```python
from build123d import *

# Parameters (mm, degrees)
ESQUISSE1_R        = 2.1
BOSS_EXTRU_1_DEPTH = 150


with BuildPart() as part:
    # Esquisse1 → Boss.-Extru.1 (new, symmetric)
    with BuildSketch(Plane.XY):
        with BuildLine():
            Line((-38.199999929, 10), (-34.639999675, 10))
            Line((-34.639999675, 10), (-32.839999603, 8.2))
            Line((-32.839999603, 8.2), (-35.499339671, 8.2))
            Line((-35.499339671, 8.2), (-35.499339671, 6.56))
            Line((-35.499339671, 6.56), (-32.839999603, 3.900660038))
            Line((-32.839999603, 3.900660038), (-27.159999603, 3.900660038))
            Line((-27.159999603, 3.900660038), (-24.500659536, 6.56))
            Line((-24.500659536, 6.56), (-24.500659536, 8.2))
            Line((-24.500659536, 8.2), (-27.159999603, 8.2))
            Line((-27.159999603, 8.2), (-25.359999532, 10))
            Line((-25.359999532, 10), (-14.640000468, 10))
            Line((-14.640000468, 10), (-12.840000397, 8.2))
            Line((-12.840000397, 8.2), (-15.499340464, 8.2))
            Line((-15.499340464, 8.2), (-15.499340464, 6.56))
            Line((-15.499340464, 6.56), (-12.840000397, 3.900660038))
            Line((-12.840000397, 3.900660038), (-7.159998809, 3.900660038))
            Line((-7.159998809, 3.900660038), (-4.500658742, 6.56))
            Line((-4.500658742, 6.56), (-4.500658742, 8.2))
            Line((-4.500658742, 8.2), (-7.159998809, 8.2))
            Line((-7.159998809, 8.2), (-5.359998738, 10))
            Line((-5.359998738, 10), (5.359998738, 10))
            Line((5.359998738, 10), (7.159998809, 8.2))
            Line((7.159998809, 8.2), (4.500658742, 8.2))
            Line((4.500658742, 8.2), (4.500658742, 6.56))
            Line((4.500658742, 6.56), (7.159998809, 3.900660038))
            Line((7.159998809, 3.900660038), (12.840000397, 3.900660038))
            Line((12.840000397, 3.900660038), (15.499340464, 6.56))
            Line((15.499340464, 6.56), (15.499340464, 8.2))
            Line((15.499340464, 8.2), (12.840000397, 8.2))
            Line((12.840000397, 8.2), (14.640000468, 10))
            Line((14.640000468, 10), (25.359999532, 10))
            Line((25.359999532, 10), (27.159999603, 8.2))
            Line((27.159999603, 8.2), (24.500659536, 8.2))
            Line((24.500659536, 8.2), (24.500659536, 6.56))
            Line((24.500659536, 6.56), (27.159999603, 3.900660038))
            Line((27.159999603, 3.900660038), (32.839999603, 3.900660038))
            Line((32.839999603, 3.900660038), (35.499339671, 6.56))
            Line((35.499339671, 6.56), (35.499339671, 8.2))
            Line((35.499339671, 8.2), (32.839999603, 8.2))
            Line((32.839999603, 8.2), (34.639999675, 10))
            Line((34.639999675, 10), (38.199999929, 10))
            ThreePointArc((38.199999929, 10), (39.47279216, 9.472792181), (39.999999929, 8.199999929))
            Line((39.999999929, 8.199999929), (39.999999787, 4.639999675))
            Line((39.999999787, 4.639999675), (38.199999716, 2.839999675))
            Line((38.199999716, 2.839999675), (38.199999821, 5.499339742))
            Line((38.199999821, 5.499339742), (36.559999821, 5.499339807))
            Line((36.559999821, 5.499339807), (33.900659754, 2.839999845))
            Line((33.900659754, 2.839999845), (33.900659641, 0))
            Line((33.900659641, 0), (33.900659754, -2.839999845))
            Line((33.900659754, -2.839999845), (36.559999821, -5.499339807))
            Line((36.559999821, -5.499339807), (38.199999821, -5.499339742))
            Line((38.199999821, -5.499339742), (38.199999716, -2.839999675))
            Line((38.199999716, -2.839999675), (39.999999787, -4.639999675))
            Line((39.999999787, -4.639999675), (39.999999929, -8.199999929))
            ThreePointArc((39.999999929, -8.199999929), (39.47279216, -9.472792181), (38.199999929, -10))
            Line((38.199999929, -10), (34.639999675, -10))
            Line((34.639999675, -10), (32.839999603, -8.2))
            Line((32.839999603, -8.2), (35.499339671, -8.2))
            Line((35.499339671, -8.2), (35.499339671, -6.56))
            Line((35.499339671, -6.56), (32.839999603, -3.900660038))
            Line((32.839999603, -3.900660038), (27.159999603, -3.900660038))
            Line((27.159999603, -3.900660038), (24.500659536, -6.56))
            Line((24.500659536, -6.56), (24.500659536, -8.2))
            Line((24.500659536, -8.2), (27.159999603, -8.2))
            Line((27.159999603, -8.2), (25.359999532, -10))
            Line((25.359999532, -10), (14.640000468, -10))
            Line((14.640000468, -10), (12.840000397, -8.2))
            Line((12.840000397, -8.2), (15.499340464, -8.2))
            Line((15.499340464, -8.2), (15.499340464, -6.56))
            Line((15.499340464, -6.56), (12.840000397, -3.900660038))
            Line((12.840000397, -3.900660038), (7.159998809, -3.900660038))
            Line((7.159998809, -3.900660038), (4.500658742, -6.56))
            Line((4.500658742, -6.56), (4.500658742, -8.2))
            Line((4.500658742, -8.2), (7.159998809, -8.2))
            Line((7.159998809, -8.2), (5.359998738, -10))
            Line((5.359998738, -10), (-5.359998738, -10))
            Line((-5.359998738, -10), (-7.159998809, -8.2))
            Line((-7.159998809, -8.2), (-4.500658742, -8.2))
            Line((-4.500658742, -8.2), (-4.500658742, -6.56))
            Line((-4.500658742, -6.56), (-7.159998809, -3.900660038))
            Line((-7.159998809, -3.900660038), (-12.840000397, -3.900660038))
            Line((-12.840000397, -3.900660038), (-15.499340464, -6.56))
            Line((-15.499340464, -6.56), (-15.499340464, -8.2))
            Line((-15.499340464, -8.2), (-12.840000397, -8.2))
            Line((-12.840000397, -8.2), (-14.640000468, -10))
            Line((-14.640000468, -10), (-25.359999532, -10))
            Line((-25.359999532, -10), (-27.159999603, -8.2))
            Line((-27.159999603, -8.2), (-24.500659536, -8.2))
            Line((-24.500659536, -8.2), (-24.500659536, -6.56))
            Line((-24.500659536, -6.56), (-27.159999603, -3.900660038))
            Line((-27.159999603, -3.900660038), (-32.839999603, -3.900660038))
            Line((-32.839999603, -3.900660038), (-35.499339671, -6.56))
            Line((-35.499339671, -6.56), (-35.499339671, -8.2))
            Line((-35.499339671, -8.2), (-32.839999603, -8.2))
            Line((-32.839999603, -8.2), (-34.639999675, -10))
            Line((-34.639999675, -10), (-38.199999929, -10))
            ThreePointArc((-38.199999929, -10), (-39.47279216, -9.472792181), (-39.999999929, -8.199999929))
            Line((-39.999999929, -8.199999929), (-39.999999787, -4.639999675))
            Line((-39.999999787, -4.639999675), (-38.199999716, -2.839999675))
            Line((-38.199999716, -2.839999675), (-38.199999821, -5.499339742))
            Line((-38.199999821, -5.499339742), (-36.559999821, -5.499339807))
            Line((-36.559999821, -5.499339807), (-33.900659754, -2.839999845))
            Line((-33.900659754, -2.839999845), (-33.900659641, 0))
            Line((-33.900659641, 0), (-33.900659754, 2.839999845))
            Line((-33.900659754, 2.839999845), (-36.559999821, 5.499339807))
            Line((-36.559999821, 5.499339807), (-38.199999821, 5.499339742))
            Line((-38.199999821, 5.499339742), (-38.199999716, 2.839999675))
            Line((-38.199999716, 2.839999675), (-39.999999787, 4.639999675))
            Line((-39.999999787, 4.639999675), (-39.999999929, 8.199999929))
            ThreePointArc((-39.999999929, 8.199999929), (-39.47279216, 9.472792181), (-38.199999929, 10))
        make_face()
        with Locations((-29.999999603, 0)):
            Circle(ESQUISSE1_R, mode=Mode.SUBTRACT)
        with Locations((-9.999999603, 0)):
            Circle(ESQUISSE1_R, mode=Mode.SUBTRACT)
        with Locations(Location((29.999999603, 0, 0), (0, 0, 180))):
            Circle(ESQUISSE1_R, mode=Mode.SUBTRACT)
        with Locations(Location((9.999999603, 0, 0), (0, 0, 180))):
            Circle(ESQUISSE1_R, mode=Mode.SUBTRACT)
        Polygon((-38.199999929, 8.2), (-38.199999864, 6.569339742), (-37.629999799, 6.569339742), (-36.569339648, 7.629999935), (-36.569339648, 8.2), align=None, mode=Mode.SUBTRACT)
        Polygon((-17.3, 6.239339079), (-17.3, 8.2), (-22.7, 8.2), (-22.7, 6.239339079), (-26.099339368, 2.839999845), (-26.099339368, -2.839999845), (-22.7, -6.239339079), (-22.7, -8.2), (-17.3, -8.2), (-17.3, -6.239339079), (-13.900660632, -2.839999845), (-13.900660632, 2.839999845), align=None, mode=Mode.SUBTRACT)
        Polygon((-6.099339678, -2.840000949), (-6.099339678, 2.840000949), (-2.700001413, 6.239339079), (-2.700001413, 8.2), (2.700001413, 8.2), (2.700001413, 6.239339079), (6.099339678, 2.840000949), (6.099339678, -2.840000949), (2.700001413, -6.239339079), (2.700001413, -8.2), (-2.700001413, -8.2), (-2.700001413, -6.239339079), align=None, mode=Mode.SUBTRACT)
        Polygon((-36.569339648, -7.629999935), (-36.569339648, -8.2), (-38.199999929, -8.2), (-38.199999864, -6.569339742), (-37.629999799, -6.569339742), align=None, mode=Mode.SUBTRACT)
        Polygon((36.569339648, 8.2), (38.199999929, 8.2), (38.199999864, 6.569339742), (37.629999799, 6.569339742), (36.569339648, 7.629999935), align=None, mode=Mode.SUBTRACT)
        Polygon((36.569339648, -8.2), (38.199999929, -8.2), (38.199999864, -6.569339742), (37.629999799, -6.569339742), (36.569339648, -7.629999935), align=None, mode=Mode.SUBTRACT)
        Polygon((13.900660632, -2.839999845), (17.3, -6.239339079), (17.3, -8.2), (22.7, -8.2), (22.7, -6.239339079), (26.099339368, -2.839999845), (26.099339368, 2.839999845), (22.7, 6.239339079), (22.7, 8.2), (17.3, 8.2), (17.3, 6.239339079), (13.900660632, 2.839999845), align=None, mode=Mode.SUBTRACT)
    extrude(amount=BOSS_EXTRU_1_DEPTH, both=True)


solid = part.part
```
Part model, mm, in its own coordinate system. A direction names the side the tool comes from. Round coordinates to 2 decimals unless told otherwise and drop trailing zeros. Write each loop counter-clockwise with the first axis right and the second up, starting at its lowest first coordinate (ties: lowest second). Pieces come first, ordered by that corner, then holes. Notation, with made-up numbers: M 72,42 L 81,42 A27 cw 81,74 Z; hole C -14,30.5 d11. An arc over 180 degrees is marked long. One line per question, with ' | ' between items.
(1) 3-axis set-ups, long thin cutter, end or side, ignore diameter. For faces 1 (the face through (20, 8.2, 2)), 2 (the face through (-30, -3.901, 2)), 3 (the face through (20, -10, 2)), 4 (the face through (30, 3.901, 2)): which of +Z, -Z, +X, -X, +Y, -Y reach the whole face in a straight line?
Answer key:
face 1: +Z, -Z | face 2: +Z, -Z, -Y | face 3: +Z, -Z, +X, -X, -Y | face 4: +Z, -Z, +Y
(2) Saw through at A-A on x = 0. Write the cut outline in (y, z).
Answer key:
outline: M -10,-150 L -8.2,-150 L -8.2,150 L -10,150 Z; M 8.2,-150 L 10,-150 L 10,150 L 8.2,150 Z
(3) Probe line 1 along Y through (x, z) = (-10, 35); line 2 along Y through (x, z) = (-25, 102.5); line 3 along X through (y, z) = (3.25, -99). List the from-to ranges inside material, lowest first.
Answer key:
line 1: y = -3.9 to -2.1, 2.1 to 3.9 | line 2: y = -10 to -8.2, -6.06 to -3.94, 3.94 to 6.06, 8.2 to 10 | line 3: x = -38.61 to -38.2, -34.31 to -25.69, -14.31 to -5.69, 5.69 to 14.31, 25.69 to 34.31, 38.2 to 38.61
(4) Pin check, flat tips, straight feed: pin 1 (3 mm diameter, centred on x = 29, z = -5.5, fed in from +Y); pin 2 (2 mm diameter, centred on x = -11, y = -6.5, fed in from -Z); pin 3 (2 mm diameter, centred on x = 13.5, z = -21, fed in from +Y); pin 4 (1 mm diameter, centred on y = -1.5, z = -101, fed in from -X). Stop position of each tip, or through.
Answer key:
pin 1: stops at y = 3.9 | pin 2: passes through | pin 3: stops at y = 9.86 | pin 4: stops at x = -33.9
(5) Two-plate mould, pull along Y, no slides. Class faces 5 (the face through (26.099, 0, 2)), 6 (the face through (-20, -10, 2)), 7 (the face through (10, 3.901, 2)): released by +Y, released by -Y, zero draft, split by the parting line, or undercut.
Answer key:
face 5: undercut | face 6: released by -Y | face 7: released by +Y
(6) Saw through at B-B on z = -56.5. Count the separate pieces of the cut face and the enclosed holes in it, then the cut area to 3 significant figures.
Answer key:
separate pieces: 1 | enclosed holes: 11 | area: 546 mm^2
